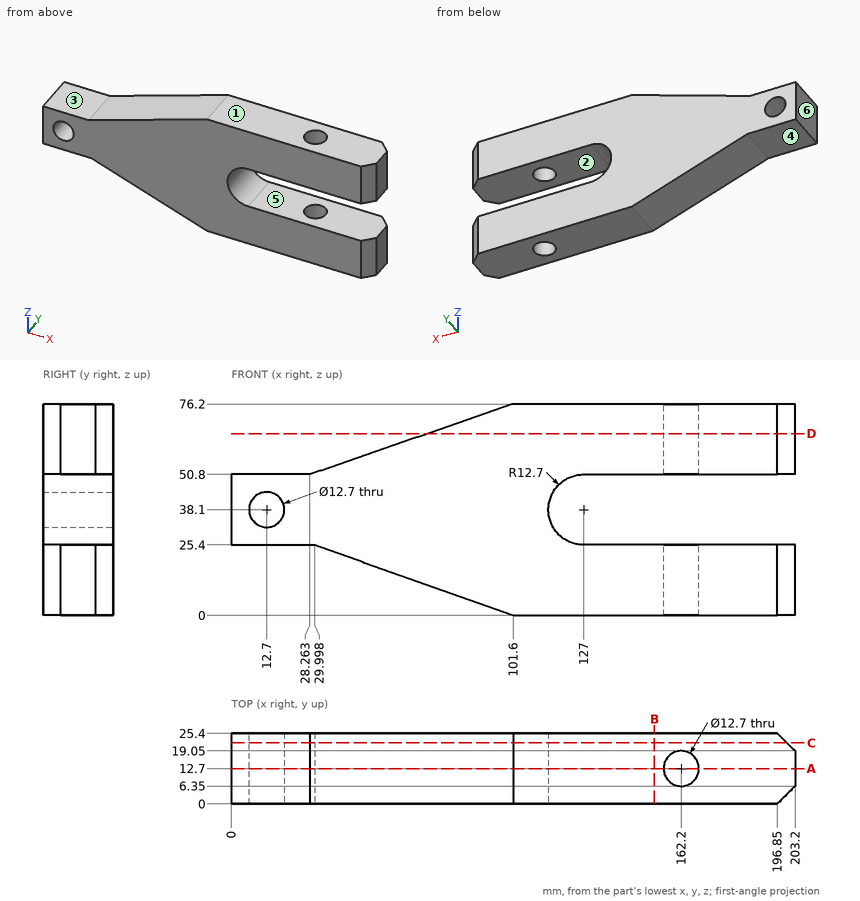
Design review of the part shown in the three views and the two pictorial views. Dimensions are in mm from the part's minimum x, y and z. A direction names the side the tool comes from. Round coordinates to 2 decimals unless told otherwise and drop trailing zeros. Write each loop counter-clockwise with the first axis right and the second up, starting at its lowest first coordinate (ties: lowest second). Pieces come first, ordered by that corner, then holes.
1) For line 1 along Z through (x, y) = (12.7, 15.5); line 2 along Y through (x, z) = (162.2, 7.5); line 3 along Z through (x, y) = (180.5, 24.5), list the stretches that pass through material, from the lowest coordinate up.
Answer below:
line 1: z = 25.4 to 31.75, 44.45 to 50.8
line 2: y = 0 to 6.35, 19.05 to 25.4
line 3: z = 0 to 25.4, 50.8 to 76.2
2) Take a section at D-D on z = 65.5. Give the boundary of the cut face in (x, y), then the cut area to 3 significant figures.
Answer below:
outline: (70.71, 0) - (196.85, 0) - (203.2, 6.35) - (203.2, 19.05) - (196.85, 25.4) - (70.71, 25.4) - close; hole circle Ø12.7 at (162.2, 12.7)
area: 3,200 mm2
3) Machinability: for the marked faces 1, 2 and 3, which of the approach directions +Z, -Z, +X, -X, +Y, -Y give a long, thin tool a straight path to every point of the face, cutting with its end or side? Answer none if there is none.
Answer below:
face 1: +Z, +X, -X, +Y, -Y
face 2: +X, +Y, -Y
face 3: +Z, -X, +Y, -Y
4) Insertion check: pin 1 Ø10 at (y, z) = (14.5, 36) entering from +X; pin 2 Ø7.5 at (x, y) = (20.5, 13) entering from +Z. Each pin has a flat end and moves straight along its axis. Give the tip position at first contact, or say it passes through.
Answer below:
pin 1: stops at x = 116.47
pin 2: stops at z = 50.8
5) Mouldability with a two-part tool opening along Z and no side actions: class the marked faces 4, 5 and 6 as +Z half, -Z half, draft (parallel to the pull), parting line (faces both ways), or undercut.
Answer below:
face 4: -Z half
face 5: undercut
face 6: draft
6) Take a section at B-B on x = 152.5. Give the boundary of the cut face in (y, z).
Answer below:
outline: (0, 0) - (25.4, 0) - (25.4, 25.4) - (0, 25.4) - close; (0, 50.8) - (25.4, 50.8) - (25.4, 76.2) - (0, 76.2) - close
7) Take a section at A-A on y = 12.7. Give the boundary of the cut face in (x, z), then the cut area to 3 significant figures.
Answer below:
outline: (0, 25.4) - (30, 25.4) - (101.6, 0) - (155.85, 0) - (155.85, 25.4) - (127, 25.4) arc R12.7 cw to (127, 50.8) - (155.85, 50.8) - (155.85, 76.2) - (101.6, 76.2) - (28.26, 50.8) - (0, 50.8) - close; (168.55, 0) - (203.2, 0) - (203.2, 25.4) - (168.55, 25.4) - close; (168.55, 50.8) - (203.2, 50.8) - (203.2, 76.2) - (168.55, 76.2) - close; hole circle Ø12.7 at (12.7, 38.1)
area: 9,200 mm2
8) Take a section at C-C on y = 22. Give the boundary of the cut face in (x, z), then the cut area to 3 significant figures.
Answer below:
outline: (0, 25.4) - (30, 25.4) - (101.6, 0) - (200.25, 0) - (200.25, 25.4) - (127, 25.4) arc R12.7 cw to (127, 50.8) - (200.25, 50.8) - (200.25, 76.2) - (101.6, 76.2) - (28.26, 50.8) - (0, 50.8) - close; hole circle Ø12.7 at (12.7, 38.1)
area: 9,700 mm2
